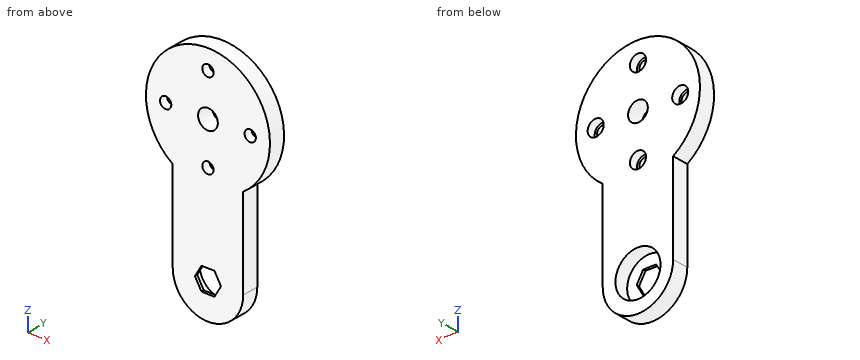
from build123d import *

# Parameters (mm, degrees)
BOSS_EXTRUDE1_DEPTH = 6
SKETCH2_R           = 2.85
CUT_EXTRUDE1_DEPTH  = 3
SKETCH3_R           = 2
SKETCH3_R_2         = 3.5
CUT_EXTRUDE2_DEPTH  = 76.524830354
SKETCH4_R           = 8
CUT_EXTRUDE3_DEPTH  = 5
SKETCH5_R           = 3.5
CUT_EXTRUDE4_DEPTH  = 76.524830354
CUT_EXTRUDE5_DEPTH  = 3


with BuildPart() as part:
    # Sketch1 → Boss-Extrude1 (new body)
    with BuildSketch(Plane(origin=(0, 0, 0), x_dir=(1, 0, 0), z_dir=(0, 1, 0))):
        with BuildLine():
            Line((-12.5, 0), (-12.5, -31.89613301))
            ThreePointArc((-12.5, -31.89613301), (0, -72), (12.5, -31.89613301))
            Line((12.5, -31.89613301), (12.5, 0))
            ThreePointArc((12.5, 0), (0, 12.5), (-12.5, 0))
        make_face()
    extrude(amount=BOSS_EXTRUDE1_DEPTH)

    # Sketch2 → Cut-Extrude1 (cut)
    with BuildSketch(Plane(origin=(0, 6, 0), x_dir=(1, 0, 0), z_dir=(0, 1, 0))):
        with Locations(Location((0, -35, 0), (0, 0, 270))):
            Circle(SKETCH2_R)
        with Locations(Location((15, -50, 0), (0, 0, 270))):
            Circle(SKETCH2_R)
        with Locations(Location((0, -65, 0), (0, 0, 270))):
            Circle(SKETCH2_R)
        with Locations(Location((-15, -50, 0), (0, 0, 270))):
            Circle(SKETCH2_R)
    extrude(amount=-CUT_EXTRUDE1_DEPTH, mode=Mode.SUBTRACT)

    # Sketch3 → Cut-Extrude2 (cut, through all)
    with BuildSketch(Plane(origin=(0, 6, 0), x_dir=(1, 0, 0), z_dir=(0, 1, 0))):
        with Locations(Location((0, -35, 0), (0, 0, 270))):
            Circle(SKETCH3_R)
        with Locations(Location((15, -50, 0), (0, 0, 270))):
            Circle(SKETCH3_R)
        with Locations(Location((0, -65, 0), (0, 0, 270))):
            Circle(SKETCH3_R)
        with Locations(Location((-15, -50, 0), (0, 0, 270))):
            Circle(SKETCH3_R)
        with Locations(Location((0, -50, 0), (0, 0, 270))):
            Circle(SKETCH3_R_2)
    extrude(amount=-CUT_EXTRUDE2_DEPTH, mode=Mode.SUBTRACT)

    # Sketch4 → Cut-Extrude3 (cut)
    with BuildSketch(Plane(origin=(0, 6, 0), x_dir=(1, 0, 0), z_dir=(0, 1, 0))):
        with Locations(Location((0, 0, 0), (0, 0, 270))):
            Circle(SKETCH4_R)
    extrude(amount=-CUT_EXTRUDE3_DEPTH, mode=Mode.SUBTRACT)

    # Sketch5 → Cut-Extrude4 (cut, through all)
    with BuildSketch(Plane(origin=(0, 6, 0), x_dir=(1, 0, 0), z_dir=(0, 1, 0))):
        with Locations(Location((0, 0, 0), (0, 0, 270))):
            Circle(SKETCH5_R)
    extrude(amount=-CUT_EXTRUDE4_DEPTH, mode=Mode.SUBTRACT)

    # Sketch6 → Cut-Extrude5 (cut)
    with BuildSketch(Plane.XZ):
        Polygon((4.618802154, 0), (2.309401077, 4), (-2.309401077, 4), (-4.618802154, 0), (-2.309401077, -4), (2.309401077, -4), align=None)
    extrude(amount=-CUT_EXTRUDE5_DEPTH, mode=Mode.SUBTRACT)


solid = part.part
Model file for the job. Use its own axes, mm. Give positions to 0.01 mm unless a question says otherwise; leave off trailing zeros. Order: outer loops, then holes, each group sorted by start corner. A loop starts at its lowest first (then second) coordinate and runs counter-clockwise, first axis right, second up. Notation, with made-up numbers: M 28.25,2.5 L 63.25,2.5 A27 ccw 63.25,19.5 Z; hole C 20.5,73 d10. An arc over 180 degrees is marked long. Put each result on its own line as item: value. Start each with the question number.
(1) Band-saw the part on D-D on x = -15. Give the cut face in (y, z), then the cut area to 3 significant figures.
(2) Drill centre lines: L1, parallel to X at y = 3.9, z = 50; L2, parallel to X at y = 0.85, z = 50; L3, parallel to Z at x = 2, y = 4.6. Where is each one in solid material? Low to high. Write a range as [from, to].
(3) Band-saw the part on B-B on z = 50. Give the cut face in (x, y).
(4) Pin check, flat tips, straight feed: pin 1 Ø4.5 at (x, z) = (0, 65) entering from +Y; pin 2 Ø2 at (x, y) = (-17.5, 2.5) entering from +Z; pin 3 Ø3 at (x, y) = (-14.5, 3) entering from -Z. Stop position of each tip, or through.
(5) Band-saw the part on A-A on x = 0. Count the separate pieces of the cut face and the enclosed holes in it, then the cut area to 3 significant figures.
(6) Band-saw the part on C-C on y = 4.3. Give the cut face in (x, z).
Results below:
1. outline: M 0,33.91 L 6,33.91 L 6,47.15 L 3,47.15 L 3,48 L 0,48 Z; M 0,52 L 3,52 L 3,52.85 L 6,52.85 L 6,66.09 L 0,66.09 Z
1. area: 164 mm2
2. L1: x = [-22, -17.85], [-12.15, -3.5], [3.5, 12.15], [17.85, 22]
2. L2: x = [-22, -17], [-13, -3.5], [3.5, 13], [17, 22]
2. L3: z = [-12.34, -7.75], [7.75, 32.97], [37.03, 47.13], [52.87, 62.97], [67.03, 71.91]
3. outline: M -22,0 L -17,0 L -17,3 L -17.85,3 L -17.85,6 L -22,6 Z; M -13,0 L -3.5,0 L -3.5,6 L -12.15,6 L -12.15,3 L -13,3 Z; M 3.5,0 L 13,0 L 13,3 L 12.15,3 L 12.15,6 L 3.5,6 Z; M 17,0 L 22,0 L 22,6 L 17.85,6 L 17.85,3 L 17,3 Z
4. pin 1: stops at y = 3
4. pin 2: stops at z = 64.55
4. pin 3: stops at z = 32.25
5. separate pieces: 5
5. enclosed holes: 0
5. area: 319 mm2
6. outline: M -12.5,0 A12.5 ccw 12.5,0 L 12.5,31.9 A22 ccw long -12.5,31.9 Z; hole C -15,50 d5.7; hole C 0,0 d16; hole C 0,50 d7; hole C 0,35 d5.7; hole C 0,65 d5.7; hole C 15,50 d5.7
